Part model, mm, in its own coordinate system. A direction names the side the tool comes from. Give positions to 0.01 mm unless a question says otherwise; leave off trailing zeros. Loops run counter-clockwise (first coordinate to the right, second up) from the corner with the lowest first, then second, coordinate; pieces in that order, holes last. Notation, with made-up numbers: (-34, -36.5) -> (19, -36.5) arc R14 cw to (19, -30.5) -> close; hole circle Ø11 at (39, 43). An arc over 180 degrees is marked (long way). One line per question, with ' | ' between items.
Autodesk Inventor part; units mm, degrees
ref_plane "YZ Plane" through (0, 0, 0) normal (1, 0, 0) x (0, 1, 0)
ref_plane "XZ Plane" through (0, 0, 0) normal (0, 1, 0) x (-1, 0, 0)
ref_plane "XY Plane" through (0, 0, 0) normal (0, 0, 1) x (1, 0, 0)
sketch "Эскиз1" plane through (0, 0, 0) normal (0, 0, 1) x (1, 0, 0)
  line L0 (0, 0) -> (-36, 0)
  line L1 (-36, 0) -> (-36, 6)
  line L2 (-36, 6) -> (-28, 6)
  arc A0 (0, 34) -> (-28, 6) centre (0, 6) ccw
  line L3 (0, 34) -> (0, 0) construction
  line L4 (-28, 6) -> (-28, 13.1241) construction
  circle A1 centre (0, 6) radius 4.75
  circle A2 centre (0, 25.75) radius 3.5
  line L5 (-3.493, 25.9715) -> (-4.7405, 6.3006)
  line L6 (3.493, 25.9715) -> (4.7405, 6.3006)
  line L7 (0, 0) -> (36, 0)
  line L8 (36, 0) -> (36, 6)
  line L9 (36, 6) -> (28, 6)
  arc A3 (28, 6) -> (0, 34) centre (0, 6) ccw
  line L10 (28, 6) -> (28, 13.1241) construction
  dimension "d0" = 8
  dimension "d1" = 6
  dimension "d2" = 28
  dimension "d3" = 7
  dimension "d4" = 9.5
  dimension "d5" = 19.75
extrude "Выдавливание1" add sketch "Эскиз1" along normal blind 170
sketch "Эскиз2" plane through (0, 0, 0) normal (0, 0, -1) x (-1, 0, 0)
  line L0 (-36, 6) -> (-28, 6)
  line L1 (-36, 0) -> (-36, 6)
  line L2 (36, 0) -> (-36, 0)
  line L3 (36, 6) -> (36, 0)
  line L4 (28, 6) -> (36, 6)
  arc A0 (28, 6) -> (-28, 6) centre (0, 6) ccw
  line L5 (-3.493, 25.9715) -> (-4.7405, 6.3006)
  arc A1 (3.493, 25.9715) -> (-3.493, 25.9715) centre (0, 25.75) ccw
  line L6 (4.7405, 6.3006) -> (3.493, 25.9715)
  arc A2 (-4.7405, 6.3006) -> (4.7405, 6.3006) centre (0, 6) ccw
  point P0 (0, 0)
extrude "Выдавливание2" add sketch "Эскиз2" against normal blind 167.5 contours A1 L6 A2 L5
sketch "Эскиз3" plane through (28, 6, 0) normal (0, 1, 0) x (1, 0, 0)
  line L0 (-64, 0) -> (8, 0)
  line L1 (8, 0) -> (8, -170)
  line L2 (-64, -170) -> (8, -170)
  line L3 (-64, 0) -> (-64, -170)
  line L4 (-28, 0) -> (-28, -85) construction
  line L5 (-28, -85) -> (14.415, -85) construction
  point P0 (-60, -166)
  point P1 (8, -85)
  point P2 (4, -166)
  point P3 (-60, -4)
  point P4 (4, -4)
  dimension "d10" = 4
  dimension "d11" = 4
hole "Отверстие1" at (-32, 6, 166) at (32, 6, 166) at (-32, 6, 4) at (32, 6, 4) direction (0, -1, 0) diameter 3.4 depth 6 countersink diameter 6.6 countersink angle 90
properties part number "вал форточка"
1) Saw through at A-A (z = 4). Give the cut face in (x, y), and give its area (3 significant figures).
Found:
outline: (-36, 0) -> (-33.7, 0) -> (-33.7, 4.4) -> (-35.3, 6) -> (-36, 6) -> close; (-30.3, 0) -> (30.3, 0) -> (30.3, 4.4) -> (28.7, 6) -> (28, 6) arc R28 ccw to (-28, 6) -> (-28.7, 6) -> (-30.3, 4.4) -> close; (33.7, 0) -> (36, 0) -> (36, 6) -> (35.3, 6) -> (33.7, 4.4) -> close | area: 1,620 mm2
2) Saw through at D-D (x = -17.5). Give the cut face in (y, z).
Found:
outline: (0, 0) -> (27.86, 0) -> (27.86, 170) -> (0, 170) -> close
3) Pull direction Z, two halves, no side cores. Call faces 1 (the cylindrical face through (33.5, 2.2, 4.8)), 2 (the flat face through (7, 13, 170)), 3 (the flat face through (32, 6, 84)): pulls with the +Z half, pulls with the -Z half, needs draft (parallel to the pull), parting line crosses it, or undercut.
Found:
face 1: undercut | face 2: pulls with the +Z half | face 3: needs draft
4) Saw through at B-B (x = 32). Give the cut face in (y, z).
Found:
outline: (0, 0) -> (6, 0) -> (6, 0.7) -> (4.4, 2.3) -> (0, 2.3) -> close; (0, 5.7) -> (4.4, 5.7) -> (6, 7.3) -> (6, 162.7) -> (4.4, 164.3) -> (0, 164.3) -> close; (0, 167.7) -> (4.4, 167.7) -> (6, 169.3) -> (6, 170) -> (0, 170) -> close
5) Saw through at C-C (z = 123). Give the cut face in (x, y).
Found:
outline: (-36, 0) -> (36, 0) -> (36, 6) -> (28, 6) arc R28 ccw to (-28, 6) -> (-36, 6) -> close
6) Tool access for faces 4 (the cylindrical face through (-30.5, 2.2, 4.8)), 5 (the flat face through (-32, 6, 84)), 6 (the flat face through (0, 15, 167.5)): list every direction of +Z, -Z, +X, -X, +Y, -Y with a clear straight run to the whole face (end or side of a thin tool).
Found:
face 4: +Y, -Y | face 5: +Z, -Z, -X, +Y | face 6: +Z
7) Pin check, flat tips, straight feed: P1, Ø6.5, axis at x = -32, z = 52.5, coming from the +Y side; P2, Ø1, axis at y = 18.5, z = 132.5, coming from the -X side; P3, Ø1.5, axis at x = -19.5, z = 31.5, coming from the +Y side; P4, Ø3, axis at x = 32, z = 166, coming from the +Y side. Stop position of each tip, or through.
Found:
P1: y = 6 | P2: x = -25.3 | P3: y = 26.8 | P4: through
8) Drill centre lines: line 1 (X direction, y = 2, z = 166); line 2 (Z direction, x = -32, y = 1); line 3 (Z direction, x = -1.5, y = 14.5). Where is each one in solid material? Low to high.
Found:
line 1: -36 to -33.7, -30.3 to 30.3, 33.7 to 36 | line 2: 0 to 2.3, 5.7 to 164.3, 167.7 to 170 | line 3: 0 to 167.5
